CAD build for the part. Positions are in the model's coordinates, mm. A direction names the side the tool comes from. Give positions to 0.01 mm unless a question says otherwise; leave off trailing zeros. Write each loop counter-clockwise with the first axis right and the second up, starting at its lowest first coordinate (ties: lowest second). Pieces come first, ordered by that corner, then holes. Notation, with made-up numbers: (34.5, 61) -> (47.5, 61) arc R5 cw to (47.5, 68) -> close; hole circle Ø10 at (59, 86.5). An arc over 180 degrees is marked (long way). Use one line per item in the form item = value. Start each with the question number.
from build123d import *

# Parameters (mm, degrees)
BOSS_EXTRUDE1_DEPTH = 26.162
SKETCH3_R           = 1.905
CUT_EXTRUDE2_DEPTH  = 5.08
SKETCH2_R           = 2.54
CUT_EXTRUDE3_DEPTH  = 50.07790077


with BuildPart() as part:
    # Sketch1 → Boss-Extrude1 (new body)
    with BuildSketch(Plane(origin=(0, 0, 0), x_dir=(1, 0, 0), z_dir=(0, 1, 0))):
        Polygon((38.1, -12.7), (-38.1, -12.7), (-38.1, 12.7), (-33.02, 12.7), (-3.81, 0), (-3.81, -3.81), (3.81, -3.81), (3.81, 0), (33.02, 12.7), (38.1, 12.7), align=None)
    extrude(amount=BOSS_EXTRUDE1_DEPTH)

    # Sketch3 → Cut-Extrude2 (cut)
    with BuildSketch(Plane(origin=(0, 26.162, 0), x_dir=(1, 0, 0), z_dir=(0, 1, 0))):
        with Locations(Location((0, -8.89, 0), (0, 0, 270))):
            Circle(SKETCH3_R)
    extrude(amount=-CUT_EXTRUDE2_DEPTH, mode=Mode.SUBTRACT)

    # Sketch2 → Cut-Extrude3 (cut, through all)
    with BuildSketch(Plane(origin=(0, 0, 3.81), x_dir=(-1, 0, 0), z_dir=(0, 0, -1))):
        with Locations((0, 12.7)):
            Circle(SKETCH2_R)
    extrude(amount=-CUT_EXTRUDE3_DEPTH, mode=Mode.SUBTRACT)


solid = part.part
1) Pin check, flat tips, straight feed: pin 1 (8 mm diameter, centred on x = 0, y = 12.7, fed in from -Z); pin 2 (1 mm diameter, centred on x = 18.5, y = 21.5, fed in from -Z); pin 3 (1.1 mm diameter, centred on x = 0.5, z = 9, fed in from +Y). Stop position of each tip, or through.
2) Cut at C-C (y = 24). Give the cut face in (x, z) (3 decimals).
3) 3-axis set-ups, long thin cutter, end or side, ignore diameter. For faces 1 (the face through (36, 13, -12.7)), 2 (the face through (0, 21.082, 9)), 3 (the face through (18.21, 12.9, -6.26)): which of +Z, -Z, +X, -X, +Y, -Y reach the whole face in a straight line?
4) Cut at B-B (z = 8.89). Give the cut face in (x, y) (3 decimals).
5) Cut at D-D (z = -6). Give the cut face in (x, y), and give its area (3 significant figures).
6) Cut at A-A (x = 0). Give the cut face in (y, z) (3 decimals), and give its area (3 significant figures).
7) Wall check: line 1 along X through (y, z) = (22, 3.5); line 2 along X through (y, z) = (22.95, 8.89) (3 decimals); line 3 along Y through (x, z) = (0, 9.25). Give the ranges that are in metal, low to high. Write a range as from..to.
8) Two-plate mould, pull along X, no slides. Class faces 4 (the face through (-36, 13, -12.7)), 5 (the face through (38.1, 13, 0)), 6 (the face through (-3.81, 13, 2)): released by +X, released by -X, zero draft, split by the parting line, or undercut.
Final values:
q1.pin_1 = -0.08
q1.pin_2 = -6.6
q1.pin_3 = 21.08
q2.outline = (-38.1, -12.7) -> (-33.02, -12.7) -> (-3.81, 0) -> (-3.81, 3.81) -> (3.81, 3.81) -> (3.81, 0) -> (33.02, -12.7) -> (38.1, -12.7) -> (38.1, 12.7) -> (-38.1, 12.7) -> close; hole circle Ø3.81 at (0, 8.89)
q3.face_1 = -Z, +X, -X, +Y, -Y
q3.face_2 = +Y
q3.face_3 = -Z, +Y, -Y
q4.outline = (-38.1, 0) -> (38.1, 0) -> (38.1, 26.162) -> (1.905, 26.162) -> (1.905, 21.082) -> (-1.905, 21.082) -> (-1.905, 26.162) -> (-38.1, 26.162) -> close; hole circle Ø5.08 at (0, 12.7)
q5.outline = (-38.1, 0) -> (-17.61, 0) -> (-17.61, 26.16) -> (-38.1, 26.16) -> close; (17.61, 0) -> (38.1, 0) -> (38.1, 26.16) -> (17.61, 26.16) -> close
q5.area = 1,070 mm^2
q6.outline = (0, 3.81) -> (10.16, 3.81) -> (10.16, 12.7) -> (0, 12.7) -> close; (15.24, 3.81) -> (26.162, 3.81) -> (26.162, 6.985) -> (21.082, 6.985) -> (21.082, 10.795) -> (26.162, 10.795) -> (26.162, 12.7) -> (15.24, 12.7) -> close
q6.area = 168 mm^2
q7.line_1 = -38.1..-3.81, 3.81..38.1
q7.line_2 = -38.1..-1.905, 1.905..38.1
q7.line_3 = 0..10.16, 15.24..21.08
q8.face_4 = zero draft
q8.face_5 = released by +X
q8.face_6 = undercut
